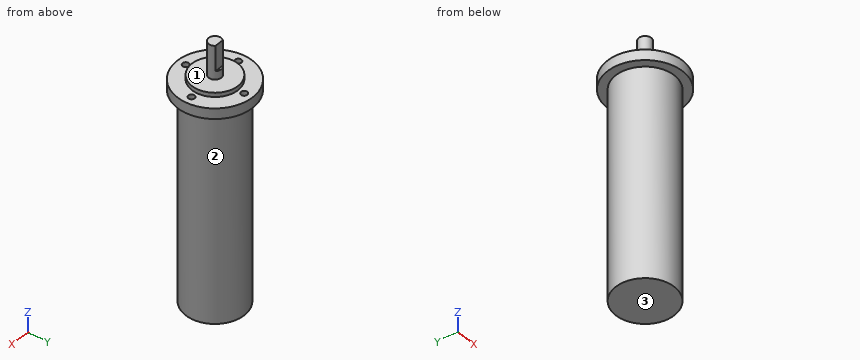
from build123d import *

# Parameters (mm, degrees)
SKETCH1_R           = 14
BOSS_EXTRUDE3_DEPTH = 100
SKETCH4_R           = 18
BOSS_EXTRUDE4_DEPTH = 5
SKETCH5_R           = 1.5
CUT_EXTRUDE2_DEPTH  = 4
SKETCH6_R           = 11
BOSS_EXTRUDE6_DEPTH = 2
SKETCH7_R           = 3
BOSS_EXTRUDE7_DEPTH = 16
SKETCH8_W           = 13.782002666
SKETCH8_H           = 7.151039119
CUT_EXTRUDE3_DEPTH  = 8


with BuildPart() as part:
    # Sketch1 → Boss-Extrude3 (new body)
    with BuildSketch(Plane.XY):
        Circle(SKETCH1_R)
    extrude(amount=BOSS_EXTRUDE3_DEPTH)

    # Sketch4 → Boss-Extrude4 (add)
    with BuildSketch(Plane.XY.offset(100)):
        Circle(SKETCH4_R)
    extrude(amount=BOSS_EXTRUDE4_DEPTH)

    # Sketch5 → Cut-Extrude2 (cut)
    with BuildSketch(Plane.XY.offset(105)):
        with Locations((0, 14)):
            Circle(SKETCH5_R)
        with Locations((14, 0)):
            Circle(SKETCH5_R)
        with Locations((0, -14)):
            Circle(SKETCH5_R)
        with Locations((-14, 0)):
            Circle(SKETCH5_R)
    extrude(amount=-CUT_EXTRUDE2_DEPTH, mode=Mode.SUBTRACT)

    # Sketch6 → Boss-Extrude6 (add)
    with BuildSketch(Plane.XY.offset(105)):
        Circle(SKETCH6_R)
    extrude(amount=BOSS_EXTRUDE6_DEPTH)

    # Sketch7 → Boss-Extrude7 (add)
    with BuildSketch(Plane.XY.offset(107)):
        Circle(SKETCH7_R)
    extrude(amount=BOSS_EXTRUDE7_DEPTH)

    # Sketch8 → Cut-Extrude3 (cut, symmetric)
    with BuildSketch(Plane(origin=(0, 0, 0), x_dir=(0, 0, -1), z_dir=(1, 0, 0))):
        with Locations((-117.891001333, 5.575519559)):
            Rectangle(SKETCH8_W, SKETCH8_H)
    extrude(amount=CUT_EXTRUDE3_DEPTH, both=True, mode=Mode.SUBTRACT)


solid = part.part
Work out the finished part from the listing and answer in its coordinate system (mm). Face numbers are marked on the shaded views. A direction names the side the tool comes from. Give positions to 0.01 mm unless a question says otherwise; leave off trailing zeros. Loops run counter-clockwise (first coordinate to the right, second up) from the corner with the lowest first, then second, coordinate; pieces in that order, holes last. Notation, with made-up numbers: (-27, -12.75) - (-1, -12.75) arc R33 ccw to (-1, 26.25) - close; hole circle Ø11 at (34, -37.5). An arc over 180 degrees is marked (long way). Answer in a Markdown table with one row per item. Add a question column.
Q1. The part is cut by section C-C (z = 17). Determine the outline of the cut face in (x, y), and give its area (3 significant figures).
Q2. A tool of negligible diameter and unlimited length cuts with its end or side. For the marked faces 1, 2 and 3, from which of +Z, -Z, +X, -X, +Y, -Y can it reach the whole face along a straight path? Write none if from no direction.
Q3. The part is cut by section D-D (y = 5.5). Determine the outline of the cut face in (x, z), and give its area (3 significant figures).
Q4. Each of these flat-tipped pins is pushed along its axis until it touches: P1, Ø1, axis at x = -9, y = 12.5, coming from the +Z side; P2, Ø0.9, axis at x = 14, y = 0.5, coming from the +Z side; P3, Ø6, axis at x = -3.5, z = 91.5, coming from the +Y side; P4, Ø5, axis at x = 0, y = 14, coming from the -Z side. Where does it stop, or does it pass through?
Q5. Consider line 1 along Y through (x, z) = (0, 103.2); line 2 along Z through (x, y) = (-12, -2); line 3 along Z through (x, y) = (10.5, 10). Determine where each line is inside the solid, lowest interval first.
Q6. The part is cut by section A-A (x = 0). Determine the outline of the cut face in (y, z), and give its area (3 significant figures).
Q7. The part is cut by section B-B (y = 0). Determine the outline of the cut face in (x, z).
Solution:
| question | item | result |
|---|---|---|
| 1 | outline | circle Ø28 at (0, 0) |
| 1 | area | 616 mm² |
| 2 | face 1 | +Z |
| 2 | face 2 | -Z |
| 2 | face 3 | -Z, +X, -X, +Y, -Y |
| 3 | outline | (-17.14, 100) - (-12.87, 100) - (-12.87, 0) - (12.87, 0) - (12.87, 100) - (17.14, 100) - (17.14, 105) - (9.53, 105) - (9.53, 107) - (-9.53, 107) - (-9.53, 105) - (-17.14, 105) - close |
| 3 | area | 2,780 mm² |
| 4 | P1 | stops at z = 105 |
| 4 | P2 | stops at z = 101 |
| 4 | P3 | stops at y = 13.99 |
| 4 | P4 | stops at z = 0 |
| 5 | line 1 | y = -18 to -15.5, -12.5 to 12.5, 15.5 to 18 |
| 5 | line 2 | z = 0 to 105 |
| 5 | line 3 | z = 100 to 105 |
| 6 | outline | (-18, 100) - (-14, 100) - (-14, 0) - (14, 0) - (14, 100) - (18, 100) - (18, 105) - (15.5, 105) - (15.5, 101) - (12.5, 101) - (12.5, 105) - (11, 105) - (11, 107) - (3, 107) - (3, 111) - (2, 111) - (2, 123) - (-3, 123) - (-3, 107) - (-11, 107) - (-11, 105) - (-12.5, 105) - (-12.5, 101) - (-15.5, 101) - (-15.5, 105) - (-18, 105) - close |
| 6 | area | 3,080 mm² |
| 7 | outline | (-18, 100) - (-14, 100) - (-14, 0) - (14, 0) - (14, 100) - (18, 100) - (18, 105) - (15.5, 105) - (15.5, 101) - (12.5, 101) - (12.5, 105) - (11, 105) - (11, 107) - (3, 107) - (3, 123) - (-3, 123) - (-3, 107) - (-11, 107) - (-11, 105) - (-12.5, 105) - (-12.5, 101) - (-15.5, 101) - (-15.5, 105) - (-18, 105) - close |
